Check sheet for the modelled part. Datum: model origin and axes. Units: mm. A direction names the side the tool comes from. Round coordinates to 2 decimals unless told otherwise and drop trailing zeros. Order: outer loops, then holes, each group sorted by start corner. A loop starts at its lowest first (then second) coordinate and runs counter-clockwise, first axis right, second up. Notation, with made-up numbers: M 6,24.25 L 57,24.25 A16 ccw 57,55.25 Z; hole C 50.5,-22.5 d3. An arc over 180 degrees is marked long. One line per item, written item: value. Start each with the question number.
(1) Cross-section at B-B, the plane z = 12.7. Count the separate pieces of the cut face and the enclosed holes in it, and give its area (3 significant figures).
(2) Depth check by flat-ended pin: pin 1 Ø8.5 at (y, z) = (68.78, 12.7) entering from -X. Enter the tip coordinate at first touch or a pass-through.
(3) Release check for a two-part mould opening along Y. For faces 1 (the face through (7, 137, 25.4)), 2 (the face through (18.363, 147.909, 11.484)), 3 (the face through (18.363, 91.004, 12.84)) record: released by +Y, released by -Y, zero draft, split by the parting line, or undercut.
(4) Cross-section at A-A, the plane y = 34. Enter the section's corners in (x, z) (3 decimals), and give its area (3 significant figures).
(5) Access from +Z, -Z, +X, -X, +Y, -Y to the whole of each face (thin tool, end or side, straight path). Record for faces 4 (the face through (0, 137, 13)), 5 (the face through (10.4, 20.7, 1.6)).
(6) Thickness scan on L1, parallel to Z at x = 0.75, y = 228.5 (3 decimals); L2, parallel to X at y = 218, z = 22; L3, parallel to Z at x = -0.75, y = -4.5. Record the ranges inside material, lowest first.
from build123d import *

# Parameters (mm, degrees)
F0_W     = 25.4
F0_H     = 304.8
F1_DEPTH = 25.4
F2_W     = 16.753317
F2_H     = 19.05
F3_DEPTH = 304.8
F5_D     = 6.35
F7_D     = 6.35


with BuildPart() as f1:
    # F0 (on Top) → F1 (new body)
    with BuildSketch(Plane.XY):
        with Locations((7.228317, 134.828891)):
            Rectangle(F0_W, F0_H)
    extrude(amount=F1_DEPTH)

    # F2 (on face) → F3 (cut)
    with BuildSketch(Plane(origin=(0, 287.228891, 0), x_dir=(-1, 0, 0), z_dir=(0, 1, 0))):
        with Locations((-8.376658, 12.7)):
            Rectangle(F2_W, F2_H)
    extrude(amount=-F3_DEPTH, mode=Mode.SUBTRACT)

    # F5 (through all)
    with Locations(Plane(origin=(-5.471683, 0, 0), x_dir=(0, -1, 0), z_dir=(-1, 0, 0))):
        with Locations((-271.976191, 12.7), (-17.976191, 12.7), (-43.376191, 12.7), (-68.776191, 12.7), (-94.176191, 12.7), (-119.576191, 12.7), (-144.976191, 12.7), (-170.376191, 12.7), (-195.776191, 12.7), (-221.176191, 12.7), (-246.576191, 12.7), (7.423809, 12.7)):
            Hole(F5_D / 2)

    # F7 (through all)
    with Locations(Plane.XY.offset(25.4)):
        with Locations((7.228317, 45.928891), (7.228317, 20.528891), (7.228317, -4.871109), (7.228317, 147.528891), (7.228317, 172.928891), (7.228317, 96.728891), (7.228317, 122.128891), (7.228317, 71.328891), (7.228317, 249.128891), (7.228317, 274.528891), (7.228317, 223.728891), (7.228317, 198.328891)):
            Hole(F7_D / 2)


solid = f1.part
Values found:
1. separate pieces: 26
1. enclosed holes: 0
1. area: 1,980 mm^2
2. pin 1: x = -5.47
3. face 1: zero draft
3. face 2: undercut
3. face 3: undercut
4. outline: M -5.472,0 L 19.928,0 L 19.928,25.4 L -5.472,25.4 Z; hole M 0,3.175 L 16.753,3.175 L 16.753,22.225 L 0,22.225 Z
4. area: 326 mm^2
5. face 4: +Y, -Y
5. face 5: +Z, -Z
6. L1: 0 to 3.175, 22.225 to 25.4
6. L2: -5.47 to 0, 16.75 to 19.93
6. L3: 0 to 11.46, 13.94 to 25.4
